```python
from build123d import *

# Parameters (mm, degrees)
SKETCH1_R           = 69.85
BOSS_EXTRUDE1_DEPTH = 12.7
CUT_EXTRUDE12_START = -10.16
CUT_EXTRUDE12_DEPTH = 10.16
SKETCH16_W          = 69.932780821
SKETCH16_H          = 69.651198358
BOSS_EXTRUDE5_DEPTH = 2.54
CUT_EXTRUDE13_DEPTH = 100.362175566
SKETCH19_R          = 3.81
SKETCH19_R_2        = 1.5875
CUT_EXTRUDE14_DEPTH = 100.362175566
FILLET27_R          = 2.54
FILLET28_R          = 2.54
FILLET31_R          = 2.54
CUT_EXTRUDE15_DEPTH = 100.362175647
CUT_EXTRUDE16_DEPTH = 100.595858501


with BuildPart() as part:
    # Sketch1 → Boss-Extrude1 (new body)
    with BuildSketch(Plane(origin=(0, 0, 0), x_dir=(1, 0, 0), z_dir=(0, 1, 0))):
        with Locations(Location((0, 0, 0), (0, 0, 270))):
            Circle(SKETCH1_R)
    extrude(amount=BOSS_EXTRUDE1_DEPTH)

    # Sketch15 → Cut-Extrude12 (cut)
    with BuildSketch(Plane(origin=(0, 12.7, 0), x_dir=(1, 0, 0), z_dir=(0, 1, 0)).offset(CUT_EXTRUDE12_START)):
        with BuildLine():
            Line((2.535588172, -66.626769527), (2.656330466, -69.799472838))
            ThreePointArc((2.656330466, -69.799472838), (49.392766771, -49.390050523), (69.799618816, -2.652491886))
            Line((69.799618816, -2.652491886), (66.626908869, -2.531924073))
            ThreePointArc((66.626908869, -2.531924073), (-47.147641009, 47.145048227), (2.535588172, -66.626769527))
        make_face()
    extrude(amount=CUT_EXTRUDE12_DEPTH, mode=Mode.SUBTRACT)

    # Sketch16 → Boss-Extrude5 (add)
    with BuildSketch(Plane(origin=(0, 2.54, 0), x_dir=(1, 0, 0), z_dir=(0, 1, 0))):
        with Locations((34.966390411, -34.825599179)):
            Rectangle(SKETCH16_W, SKETCH16_H)
    extrude(amount=-BOSS_EXTRUDE5_DEPTH)

    # Sketch18 → Cut-Extrude13 (cut, through all)
    with BuildSketch(Plane(origin=(0, 2.54, 0), x_dir=(1, 0, 0), z_dir=(0, 1, 0))):
        with BuildLine():
            Line((-2.535588172, -66.626769527), (-2.535588172, -12.444307639))
            ThreePointArc((-2.535588172, -12.444307639), (-8.966889105, -8.99360327), (-12.436709804, -2.572595822))
            Line((-12.436709804, -2.572595822), (-66.625350849, -2.572595822))
            ThreePointArc((-66.625350849, -2.572595822), (-47.133249027, -47.159436608), (-2.535588172, -66.626769527))
        make_face()
        with BuildLine():
            ThreePointArc((-12.436709804, 2.572595822), (-8.966889105, 8.99360327), (-2.535588172, 12.444307639))
            Line((-2.535588172, 12.444307639), (-2.535588172, 66.626769527))
            ThreePointArc((-2.535588172, 66.626769527), (-47.133249027, 47.159436608), (-66.625350849, 2.572595822))
            Line((-66.625350849, 2.572595822), (-12.436709804, 2.572595822))
        make_face()
        with BuildLine():
            Line((2.535588172, 66.626769527), (2.535588172, 12.444307639))
            ThreePointArc((2.535588172, 12.444307639), (8.966889105, 8.99360327), (12.436709804, 2.572595822))
            Line((12.436709804, 2.572595822), (66.625350849, 2.572595822))
            ThreePointArc((66.625350849, 2.572595822), (47.133249027, 47.159436608), (2.535588172, 66.626769527))
        make_face()
        with BuildLine():
            ThreePointArc((12.436709804, -2.572595822), (8.966889105, -8.99360327), (2.535588172, -12.444307639))
            Line((2.535588172, -12.444307639), (2.535588172, -66.626769527))
            ThreePointArc((2.535588172, -66.626769527), (47.133249027, -47.159436608), (66.625350849, -2.572595822))
            Line((66.625350849, -2.572595822), (12.436709804, -2.572595822))
        make_face()
    extrude(amount=-CUT_EXTRUDE13_DEPTH, mode=Mode.SUBTRACT)

    # Sketch19 → Cut-Extrude14 (cut, through all)
    with BuildSketch(Plane(origin=(0, 2.54, 0), x_dir=(1, 0, 0), z_dir=(0, 1, 0))):
        with Locations(Location((0, 0, 0), (0, 0, 270))):
            Circle(SKETCH19_R)
        with Locations(Location((5.828477918, 5.845842126, 0), (0, 0, 270))):
            Circle(SKETCH19_R_2)
        with Locations(Location((-5.845842126, -5.828477918, 0), (0, 0, 90))):
            Circle(SKETCH19_R_2)
        with Locations(Location((-5.864478401, 5.864478401, 0), (0, 0, 270))):
            Circle(SKETCH19_R_2)
        with Locations(Location((5.881897888, -5.847007018, 0), (0, 0, 90))):
            Circle(SKETCH19_R_2)
    extrude(amount=-CUT_EXTRUDE14_DEPTH, mode=Mode.SUBTRACT)

    # Fillet27
    fillet27_edges = [part.edges().sort_by_distance(p)[0] for p in [
        (-66.675, 2.54, 0),
    ]]
    fillet(fillet27_edges, radius=FILLET27_R)

    # Fillet28
    fillet28_edges = [part.edges().sort_by_distance(p)[0] for p in [
        (0, 2.54, -66.675),
    ]]
    fillet(fillet28_edges, radius=FILLET28_R)

    # Fillet31
    fillet31_edges = [part.edges().sort_by_distance(p)[0] for p in [
        (-49.392766771, 12.7, -49.390050523),
    ]]
    fillet(fillet31_edges, radius=FILLET31_R)

    # Sketch20 → Cut-Extrude15 (cut, through all)
    with BuildSketch(Plane(origin=(0, 2.54, 0), x_dir=(1, 0, 0), z_dir=(0, 1, 0))):
        with BuildLine():
            Line((-2.535588172, -12.444307639), (2.535588172, -12.444307639))
            Line((2.535588172, -12.444307639), (2.535588172, -66.626769527))
            ThreePointArc((2.535588172, -66.626769527), (0, -66.675), (-2.535588172, -66.626769527))
            Line((-2.535588172, -66.626769527), (-2.535588172, -12.444307639))
        make_face()
        with BuildLine():
            Line((12.436709804, -2.572595822), (12.436709804, 2.572595822))
            Line((12.436709804, 2.572595822), (66.625350849, 2.572595822))
            ThreePointArc((66.625350849, 2.572595822), (66.674996894, 0.02035079), (66.626908869, -2.531924073))
            Line((66.626908869, -2.531924073), (69.799618816, -2.652491886))
            ThreePointArc((69.799618816, -2.652491886), (69.837403568, -1.326485155), (69.85, 0))
            Line((69.85, 0), (69.932780821, 0))
            Line((69.932780821, 0), (69.932780821, -69.651198358))
            Line((69.932780821, -69.651198358), (5.266219444, -69.651198358))
            ThreePointArc((5.266219444, -69.651198358), (3.961968652, -69.737545873), (2.656330466, -69.799472838))
            Line((2.656330466, -69.799472838), (2.535588172, -66.626769527))
            ThreePointArc((2.535588172, -66.626769527), (47.133249027, -47.159436608), (66.625350849, -2.572595822))
            Line((66.625350849, -2.572595822), (12.436709804, -2.572595822))
        make_face()
    extrude(amount=-CUT_EXTRUDE15_DEPTH, mode=Mode.SUBTRACT)

    # Sketch21 → Cut-Extrude16 (cut, through all)
    with BuildSketch(Plane.XZ):
        with BuildLine():
            Line((-12.436709804, 2.572595822), (-72.625686252, 2.572595822))
            Line((-72.625686252, 2.572595822), (-72.625686252, 86.482314908))
            Line((-72.625686252, 86.482314908), (90.769446287, 86.482314908))
            Line((90.769446287, 86.482314908), (90.769446287, -81.729929128))
            Line((90.769446287, -81.729929128), (2.535588172, -81.729929128))
            Line((2.535588172, -81.729929128), (2.535588172, -12.444307639))
            ThreePointArc((2.535588172, -12.444307639), (8.966889105, -8.99360327), (12.436709804, -2.572595822))
            Line((12.436709804, -2.572595822), (12.436709804, 2.572595822))
            ThreePointArc((12.436709804, 2.572595822), (8.966889105, 8.99360327), (2.535588172, 12.444307639))
            Line((2.535588172, 12.444307639), (-2.535588172, 12.444307639))
            ThreePointArc((-2.535588172, 12.444307639), (-8.966889105, 8.99360327), (-12.436709804, 2.572595822))
        make_face()
    extrude(amount=-CUT_EXTRUDE16_DEPTH, mode=Mode.SUBTRACT)


solid = part.part
```
Part model, mm, in its own coordinate system. A direction names the side the tool comes from. Round coordinates to 2 decimals unless told otherwise and drop trailing zeros. Loops run counter-clockwise (first coordinate to the right, second up) from the corner with the lowest first, then second, coordinate; pieces in that order, holes last.
Item 1: Drop flat-ended pins along their axis: P1, Ø4, axis at y = 10, z = -18.5, coming from the -X side; P2, Ø4, axis at y = 6, z = -28.5, coming from the +X side; P3, Ø7, axis at x = 0, z = 0, coming from the -Y side; P4, Ø3, axis at x = -12.5, z = -5.5, coming from the +Y side. Give the stop position or say it passes through.
Item 2: Drill centre lines: line 1 (X direction, y = 0.95, z = 0); line 2 (Y direction, x = 0, z = -19); line 3 (X direction, y = 2.25, z = -31.5). Where is each one in solid material? Low to high.
Item 3: Cut at A-A, the plane y = 1. State how many separate pieces and enclosed holes the cut face has, then the cut area to 3 significant figures.
Item 4: Mould opens along Z. For faces 5 (the face through (-22, 0, -1)), 6 (the face through (-40, 1, -2.573)), 7 (the face through (9.04, 1.29, 8.92)) say: +Z half, -Z half, draft (parallel to the pull), parting line (faces both ways), or undercut.
Item 5: 3-axis set-ups, long thin cutter, end or side, ignore diameter. For faces 1 (the face through (-45, 2, 2.573)), 2 (the face through (2.536, 2, -48)), 3 (the face through (12.437, 1, 0)), 4 (the face through (-2.536, 1, -39)): which of +Z, -Z, +X, -X, +Y, -Y reach the whole face in a straight line?
Item 6: Cut at B-B, the plane y = 8. Give the cut face in (x, z) (3 decimals).
A:
1. P1: stops at x = -67.87
1. P2: stops at x = -59.29
1. P3: passes through
1. P4: stops at y = 2.54
2. line 1: x = -69.85 to -3.81, 3.81 to 12.44
2. line 2: y = 0 to 2.54
2. line 3: x = -62.34 to -58.76, -2.54 to 2.54
3. separate pieces: 1
3. enclosed holes: 6
3. area: 1,340 mm2
4. face 5: draft
4. face 6: undercut
4. face 7: +Z half
5. face 1: +Z, -X, +Y, -Y
5. face 2: -Z, +X, +Y, -Y
5. face 3: +Z, -Z, +X, +Y, -Y
5. face 4: +Y, -Y
6. outline: (-69.803, 2.573) arc R69.85 ccw to (2.536, -69.804) - (2.536, -66.627) arc R66.675 cw to (-66.625, 2.573) - close
